```python
from build123d import *

# Parameters (mm, degrees)
SKETCH_1_R          = 34
EXTRUDE_1_DEPTH     = 25
CUT_EXTRUDE_1_DEPTH = 25


with BuildPart() as part:
    # 草图1 → 凸台-拉伸1 (new body)
    with BuildSketch(Plane(origin=(0, 0, 0), x_dir=(1, 0, 0), z_dir=(0, 1, 0))):
        Circle(SKETCH_1_R)
    extrude(amount=EXTRUDE_1_DEPTH)

    # 草图2 → 切除-拉伸1 (cut)
    with BuildSketch(Plane.XZ):
        with BuildLine():
            add(Edge.make_bspline(
                [(0, -6.142670146), (8.892207312, -17.25267682), (0, -28.653962674)],
                knots=[0, 0, 0, 1, 1, 1], degree=2))
            add(Edge.make_bspline(
                [(0, -6.142670146), (-8.892207312, -17.25267682), (0, -28.653962674)],
                knots=[0, 0, 0, 1, 1, 1], degree=2))
        make_face()
        with BuildLine():
            add(Edge.make_bspline(
                [(-4.304164555, -3.01551155), (-17.618251974, 2.008299288), (-25.713676003, -9.971883506)],
                knots=[0, 0, 0, 1, 1, 1], degree=2))
            add(Edge.make_bspline(
                [(-4.304164555, -3.01551155), (-12.122565621, -14.905684128), (-25.713676003, -9.971883506)],
                knots=[0, 0, 0, 1, 1, 1], degree=2))
        make_face()
        with BuildLine():
            add(Edge.make_bspline(
                [(-2.660119988, 2.044337347), (-1.996471231, 16.259229872), (-15.891925746, 20.256355567)],
                knots=[0, 0, 0, 1, 1, 1], degree=2))
            add(Edge.make_bspline(
                [(-2.660119988, 2.044337347), (-16.384364896, 5.805813236), (-15.891925746, 20.256355567)],
                knots=[0, 0, 0, 1, 1, 1], degree=2))
        make_face()
        with BuildLine():
            add(Edge.make_bspline(
                [(2.660119988, 2.044337347), (16.384364896, 5.805813236), (15.891925746, 20.256355567)],
                knots=[0, 0, 0, 1, 1, 1], degree=2))
            add(Edge.make_bspline(
                [(2.660119988, 2.044337347), (1.996471231, 16.259229872), (15.891925746, 20.256355567)],
                knots=[0, 0, 0, 1, 1, 1], degree=2))
        make_face()
        with BuildLine():
            add(Edge.make_bspline(
                [(4.304164555, -3.01551155), (12.122565621, -14.905684128), (25.713676003, -9.971883506)],
                knots=[0, 0, 0, 1, 1, 1], degree=2))
            add(Edge.make_bspline(
                [(4.304164555, -3.01551155), (17.618251974, 2.008299288), (25.713676003, -9.971883506)],
                knots=[0, 0, 0, 1, 1, 1], degree=2))
        make_face()
    extrude(amount=-CUT_EXTRUDE_1_DEPTH, mode=Mode.SUBTRACT)


solid = part.part
```
Geometry check sheet. Reference: the model listing, model coordinates, mm. Round coordinates to 2 decimals unless told otherwise and drop trailing zeros. Order: outer loops, then holes, each group sorted by start corner. A loop starts at its lowest first (then second) coordinate and runs counter-clockwise, first axis right, second up. Notation, with made-up numbers: (15, 54.5) - (59, 54.5) arc R7 ccw to (59, 61.5) - close; hole circle Ø8 at (-3, -3.75). An arc over 180 degrees is marked (long way). Use a Markdown table: item, result. Add a question column.
1) Thickness scan on line 1 along Z through (x, y) = (-10, 22); line 2 along X through (y, z) = (4.75, 11.5); line 3 along Z through (x, y) = (13, 9.25). Record the ranges inside material, lowest first.
2) Gauge pin test, flat ends, axial feed: P1, Ø12, axis at y = 14, z = 15.5, coming from the +X side; P2, Ø1.5, axis at x = -12.5, z = -3, coming from the +Y side; P3, Ø5, axis at x = -7, y = 13, coming from the +Z side; P4, Ø3, axis at y = 6.5, z = 15, coming from the +X side. Record the tip position at first contact, or that the pin passes through.
3) Section check D-D (x = 30). Record the cut outline in (y, z), then the cut area to 3 significant figures.
4) Section check A-A (y = 17.75). Count the separate pieces of the cut face and the enclosed holes in it, then the cut area to 3 significant figures.
Established:
| question | item | result |
|---|---|---|
| 1 | line 1 | -32.5 to -8.97, -1.62 to 5.56, 17.71 to 32.5 |
| 1 | line 2 | -32 to -14.52, -4.32 to 4.32, 14.52 to 32 |
| 1 | line 3 | -31.42 to -10.5, -1.58 to 8.72, 19.25 to 31.42 |
| 2 | P1 | x = 32.65 |
| 2 | P2 | through |
| 2 | P3 | z = 33.7 |
| 2 | P4 | x = 31.2 |
| 3 | outline | (0, -16) - (25, -16) - (25, 16) - (0, 16) - close |
| 3 | area | 800 mm2 |
| 4 | separate pieces | 1 |
| 4 | enclosed holes | 5 |
| 4 | area | 2,960 mm2 |
